from build123d import *

# Parameters (mm, degrees)
SKETCH1_W                                       = 40
SKETCH1_H                                       = 10
BOSS_EXTRUDE1_DEPTH                             = 19.85
CSK_FOR_M3_FLAT_HEAD_MACHINE_SCREW1_D           = 3.4
CSK_FOR_M3_FLAT_HEAD_MACHINE_SCREW1_CSINK_D     = 6.3
CSK_FOR_M3_FLAT_HEAD_MACHINE_SCREW1_CSINK_ANGLE = 90
M3X0_5_TAPPED_HOLE1_D                           = 2.5
F_2_0MM_DOWEL_HOLE1_D                           = 2


with BuildPart() as part:
    # Sketch1 → Boss-Extrude1 (new body)
    with BuildSketch(Plane(origin=(0, 0, 0), x_dir=(1, 0, 0), z_dir=(0, 1, 0))):
        with Locations((20, 5)):
            Rectangle(SKETCH1_W, SKETCH1_H)
    extrude(amount=BOSS_EXTRUDE1_DEPTH)

    # CSK for M3 Flat Head Machine Screw1 (through all)
    with Locations(Plane(origin=(5, 19.85, -5), x_dir=(0, 0, 1), z_dir=(0, 1, 0))):
        with Locations((0, 0), (0, 30)):
            CounterSinkHole(CSK_FOR_M3_FLAT_HEAD_MACHINE_SCREW1_D / 2, CSK_FOR_M3_FLAT_HEAD_MACHINE_SCREW1_CSINK_D / 2, counter_sink_angle=CSK_FOR_M3_FLAT_HEAD_MACHINE_SCREW1_CSINK_ANGLE)

    # M3x0.5 Tapped Hole1 (through all)
    with Locations(Plane(origin=(20, 9.925, -10), x_dir=(-1, 0, 0), z_dir=(0, 0, -1))):
        with Locations((0, 0)):
            Hole(M3X0_5_TAPPED_HOLE1_D / 2)

    # Ø2.0mm Dowel Hole1 (through all)
    with Locations(Plane(origin=(26, 19.85, -5), x_dir=(0, 0, 1), z_dir=(0, 1, 0))):
        with Locations((0, 0)):
            Hole(F_2_0MM_DOWEL_HOLE1_D / 2)


solid = part.part
Input: part model. Units: mm. Frame: model coordinates. Give positions to 0.01 mm unless a question says otherwise; leave off trailing zeros. Order: outer loops, then holes, each group sorted by start corner. A loop starts at its lowest first (then second) coordinate and runs counter-clockwise, first axis right, second up. Notation, with made-up numbers: (38.25, -22) - (80.25, -22) arc R24 cw to (80.25, 15) - close; hole circle Ø3 at (1.25, 82.5). An arc over 180 degrees is marked (long way). Answer as a JSON object with one key per item and string values. Group by question number.
Q1. Cut plane C-C, the plane z = -5. Output: boundary loops of the cut face in (x, y) (3 decimals), then the cut area to 3 significant figures.
Q2. Cut plane D-D, the plane x = 20. Output: boundary loops of the cut face in (y, z) (3 decimals).
Q3. Mould query, pull axis X, two halves, no side actions, for faces 1 (the face through (40, 10, -5)), 2 (the face through (3.5, 9.1, -5.8)), 3 (the face through (20, 0, -5)). Classes: pulls with the +X half, pulls with the -X half, needs draft (parallel to the pull), parting line crosses it, or undercut.
Q4. Line query: probe 1 along X at (y, z) = (6, -5); probe 2 along Z at (x, y) = (35, 4.5); probe 3 along Y at (x, z) = (20, -7.5) (3 decimals). Output: solid intervals per line, ascending.
Q5. Cut plane B-B, the plane y = 15.5. Output: boundary loops of the cut face in (x, z), then the cut area to 3 significant figures.
Q6. First-contact query: pin 1 Ø2.5 at (x, z) = (26, -5) entering from -Y. Flat tip, straight axial feed; report the tip coordinate or a pass-through.
Q7. Cut plane A-A, the plane x = 26. Output: boundary loops of the cut face in (y, z), then the cut area to 3 significant figures.
Results:
{
 "1": {"outline": "(0, 0) - (3.3, 0) - (3.3, 18.4) - (1.85, 19.85) - (0, 19.85) - close; (6.7, 0) - (25, 0) - (25, 19.85) - (8.15, 19.85) - (6.7, 18.4) - close; (27, 0) - (33.3, 0) - (33.3, 18.4) - (31.85, 19.85) - (27, 19.85) - close; (36.7, 0) - (40, 0) - (40, 19.85) - (38.15, 19.85) - (36.7, 18.4) - close; hole circle Ø2.5 at (20, 9.925)", "area": "610 mm^2"},
 "2": {"outline": "(0, -10) - (8.675, -10) - (8.675, 0) - (0, 0) - close; (11.175, -10) - (19.85, -10) - (19.85, 0) - (11.175, 0) - close"},
 "3": {"face 1": "pulls with the +X half", "face 2": "undercut", "face 3": "needs draft"},
 "4": {"probe 1": "0 to 3.3, 6.7 to 25, 27 to 33.3, 36.7 to 40", "probe 2": "-10 to -6.7, -3.3 to 0", "probe 3": "0 to 8.675, 11.175 to 19.85"},
 "5": {"outline": "(0, -10) - (40, -10) - (40, 0) - (0, 0) - close; hole circle Ø3.4 at (5, -5); hole circle Ø2 at (26, -5); hole circle Ø3.4 at (35, -5)", "area": "379 mm^2"},
 "6": {"pin 1": "y = 0"},
 "7": {"outline": "(0, -10) - (19.85, -10) - (19.85, -6) - (0, -6) - close; (0, -4) - (19.85, -4) - (19.85, 0) - (0, 0) - close", "area": "159 mm^2"}
}
